Part model, mm, in its own coordinate system. A direction names the side the tool comes from. Give positions to 0.01 mm unless a question says otherwise; leave off trailing zeros. Order: outer loops, then holes, each group sorted by start corner. A loop starts at its lowest first (then second) coordinate and runs counter-clockwise, first axis right, second up. Notation, with made-up numbers: (44.5, 88.25) - (52.5, 88.25) arc R9 ccw to (52.5, 94.25) - close; hole circle Ø10 at (57.25, 55.5). An arc over 180 degrees is marked (long way). One line per item, written item: value.
```python
from build123d import *

# Parameters (mm, degrees)
SKETCH1_W                                     = 25.4
SKETCH1_H                                     = 50.8
BOSS_EXTRUDE1_DEPTH                           = 25.4
CBORE_SLOT_FOR_6_SOCKET_HEAD_CAP_SCREW1_DEPTH = 25.4
CBORE_START                                   = 16.89481
CBORE_SLOT_FOR_6_SOCKET_HEAD_CAP_SC_3_DEPTH   = 8.50519


# Read off the part's stored shape, not the designer's step: CBORE SLOT for #6 Socket Head Cap Screw1
with BuildPart() as part:
    # Sketch1 → Boss-Extrude1 (new body)
    with BuildSketch(Plane.XY):
        Rectangle(SKETCH1_W, SKETCH1_H)
    extrude(amount=BOSS_EXTRUDE1_DEPTH)

    # CBORE SLOT for _6 Socket Head Cap Sc 2 → CBORE SLOT for #6 Socket Head Cap Screw1 (cut)
    with BuildSketch(Plane.XY):
        with BuildLine():
            Line((1.89865, -17.15135), (1.89865, -8.24865))
            ThreePointArc((1.89865, -8.24865), (0, -6.35), (-1.89865, -8.24865))
            Line((-1.89865, -8.24865), (-1.89865, -17.15135))
            ThreePointArc((-1.89865, -17.15135), (0, -19.05), (1.89865, -17.15135))
        make_face()
        with BuildLine():
            ThreePointArc((1.89865, 17.15135), (0, 19.05), (-1.89865, 17.15135))
            Line((-1.89865, 17.15135), (-1.89865, 8.24865))
            ThreePointArc((-1.89865, 8.24865), (0, 6.35), (1.89865, 8.24865))
            Line((1.89865, 8.24865), (1.89865, 17.15135))
        make_face()
    extrude(amount=CBORE_SLOT_FOR_6_SOCKET_HEAD_CAP_SCREW1_DEPTH, mode=Mode.SUBTRACT)

    # CBORE SLOT for _6 Socket Head Cap Sc 3 o → CBORE SLOT for _6 Socket Head Cap Sc 3 (cut)
    # profile 1 of 2: a face of its own
    with BuildSketch(Plane.XY.offset(CBORE_START)):
        with BuildLine():
            Line((3.57251, -17.15135), (3.57251, -8.24865))
            ThreePointArc((3.57251, -8.24865), (0, -4.67614), (-3.57251, -8.24865))
            Line((-3.57251, -8.24865), (-3.57251, -17.15135))
            ThreePointArc((-3.57251, -17.15135), (0, -20.72386), (3.57251, -17.15135))
        make_face()
        with BuildLine():
            ThreePointArc((-1.89865, -8.24865), (0, -6.35), (1.89865, -8.24865))
            Line((1.89865, -8.24865), (1.89865, -17.15135))
            ThreePointArc((1.89865, -17.15135), (0, -19.05), (-1.89865, -17.15135))
            Line((-1.89865, -17.15135), (-1.89865, -8.24865))
        make_face(mode=Mode.SUBTRACT)
    # profile 2 of 2: a face of its own
    with BuildSketch(Plane.XY.offset(CBORE_START)):
        with BuildLine():
            ThreePointArc((3.57251, 17.15135), (0, 20.72386), (-3.57251, 17.15135))
            Line((-3.57251, 17.15135), (-3.57251, 8.24865))
            ThreePointArc((-3.57251, 8.24865), (0, 4.67614), (3.57251, 8.24865))
            Line((3.57251, 8.24865), (3.57251, 17.15135))
        make_face()
        with BuildLine():
            Line((-1.89865, 8.24865), (-1.89865, 17.15135))
            ThreePointArc((-1.89865, 17.15135), (0, 19.05), (1.89865, 17.15135))
            Line((1.89865, 17.15135), (1.89865, 8.24865))
            ThreePointArc((1.89865, 8.24865), (0, 6.35), (-1.89865, 8.24865))
        make_face(mode=Mode.SUBTRACT)
    extrude(amount=CBORE_SLOT_FOR_6_SOCKET_HEAD_CAP_SC_3_DEPTH, mode=Mode.SUBTRACT)


solid = part.part
```
1) Drill centre lines: line 1 along X through (y, z) = (15, 21.5); line 2 along X through (y, z) = (9.5, 5.5); line 3 along Y through (x, z) = (-0.75, 16). Where is each one in solid material? Low to high. Write a range as from..to.
Outcome:
line 1: x = -12.7..-3.57, 3.57..12.7
line 2: x = -12.7..-1.9, 1.9..12.7
line 3: y = -25.4..-18.9, -6.5..6.5, 18.9..25.4
2) Pin check, flat tips, straight feed: pin 1 (5.5 mm diameter, centred on x = 0.5, y = -15, fed in from +Z); pin 2 (12 mm diameter, centred on x = -0.5, y = 7.5, fed in from -Z). Stop position of each tip, or through.
Outcome:
pin 1: stops at z = 16.89
pin 2: stops at z = 0
3) Cut at C-C, the plane z = 4.5. Give the cut face in (x, y), then the cut area to 3 significant figures.
Outcome:
outline: (-12.7, -25.4) - (12.7, -25.4) - (12.7, 25.4) - (-12.7, 25.4) - close; hole (-1.9, -17.15) arc R1.9 ccw to (1.9, -17.15) - (1.9, -8.25) arc R1.9 ccw to (-1.9, -8.25) - close; hole (-1.9, 8.25) arc R1.9 ccw to (1.9, 8.25) - (1.9, 17.15) arc R1.9 ccw to (-1.9, 17.15) - close
area: 1,200 mm^2
4) Cut at B-B, the plane y = 9.5. Give the cut face in (x, z).
Outcome:
outline: (-12.7, 0) - (-1.9, 0) - (-1.9, 16.89) - (-3.57, 16.89) - (-3.57, 25.4) - (-12.7, 25.4) - close; (1.9, 0) - (12.7, 0) - (12.7, 25.4) - (3.57, 25.4) - (3.57, 16.89) - (1.9, 16.89) - close
5) Which spindle directions (+Z, -Z, +X, -X, +Y, -Y) get a long thin tool onto all of the face, cutting with end or side? Do faces 1 (the cylindrical face through (-0.079, -20.723, 21.088)), 2 (the flat face through (-1.899, 13, 8)), 3 (the flat face through (0, -25.4, 13)). Say none if no direction does.
Outcome:
face 1: +Z
face 2: +Z, -Z
face 3: +Z, -Z, +X, -X, -Y
6) Cut at D-D, the plane z = 22.5. Give the cut face in (x, y), then the cut area to 3 significant figures.
Outcome:
outline: (-12.7, -25.4) - (12.7, -25.4) - (12.7, 25.4) - (-12.7, 25.4) - close; hole (-3.57, -17.15) arc R3.57 ccw to (3.57, -17.15) - (3.57, -8.25) arc R3.57 ccw to (-3.57, -8.25) - close; hole (-3.57, 8.25) arc R3.57 ccw to (3.57, 8.25) - (3.57, 17.15) arc R3.57 ccw to (-3.57, 17.15) - close
area: 1,080 mm^2
7) Cut at A-A, the plane x = 0. Give the cut face in (y, z), then the cut area to 3 significant figures.
Outcome:
outline: (-25.4, 0) - (-19.05, 0) - (-19.05, 16.89) - (-20.72, 16.89) - (-20.72, 25.4) - (-25.4, 25.4) - close; (-6.35, 0) - (6.35, 0) - (6.35, 16.89) - (4.68, 16.89) - (4.68, 25.4) - (-4.68, 25.4) - (-4.68, 16.89) - (-6.35, 16.89) - close; (19.05, 0) - (25.4, 0) - (25.4, 25.4) - (20.72, 25.4) - (20.72, 16.89) - (19.05, 16.89) - close
area: 588 mm^2
8) Mould opens along Z. For faces 4 (the flat face through (-2.4, 12.8, 16.895)), 5 (the cylindrical face through (-0.04, -19.05, 8.33)) say: released by +Z, released by -Z, zero draft, split by the parting line, or undercut.
Outcome:
face 4: released by +Z
face 5: zero draft
